from build123d import *

# Parameters (mm, degrees)
F1_DEPTH = 609.6
F3_D     = 25.4


with BuildPart() as f1:
    # F0 (on Top) → F1 (new body)
    with BuildSketch(Plane.XY):
        with BuildLine():
            ThreePointArc((38.1, 25.4), (34.380256, 34.380256), (25.4, 38.1))
            Line((25.4, 38.1), (-25.4, 38.1))
            ThreePointArc((-25.4, 38.1), (-34.380256, 34.380256), (-38.1, 25.4))
            Line((-38.1, 25.4), (-38.1, -25.4))
            ThreePointArc((-38.1, -25.4), (-34.380256, -34.380256), (-25.4, -38.1))
            Line((-25.4, -38.1), (25.4, -38.1))
            ThreePointArc((25.4, -38.1), (34.380256, -34.380256), (38.1, -25.4))
            Line((38.1, -25.4), (38.1, 25.4))
        make_face()
        with BuildLine():
            ThreePointArc((25.4, 33.3375), (31.01266, 31.01266), (33.3375, 25.4))
            Line((33.3375, 25.4), (33.3375, -25.4))
            ThreePointArc((33.3375, -25.4), (31.01266, -31.01266), (25.4, -33.3375))
            Line((25.4, -33.3375), (-25.4, -33.3375))
            ThreePointArc((-25.4, -33.3375), (-31.01266, -31.01266), (-33.3375, -25.4))
            Line((-33.3375, -25.4), (-33.3375, 25.4))
            ThreePointArc((-33.3375, 25.4), (-31.01266, 31.01266), (-25.4, 33.3375))
            Line((-25.4, 33.3375), (25.4, 33.3375))
        make_face(mode=Mode.SUBTRACT)
    extrude(amount=F1_DEPTH)

    # F3 (through all)
    with Locations(Plane.YZ.offset(38.1)):
        with Locations((0, 571.5), (0, 38.1)):
            Hole(F3_D / 2)


solid = f1.part
Here's how the part is built. I have some questions about the finished solid (model axes, mm). A direction names the side the tool comes from. Coordinates: 2 decimals unless noted, no trailing zeros. Loops run counter-clockwise (first coordinate to the right, second up) from the corner with the lowest first, then second, coordinate; pieces in that order, holes last. Notation, with made-up numbers: (-21.75, 48.5) -> (37.25, 48.5) arc R13 cw to (37.25, 61.5) -> close; hole circle Ø6 at (-24, 85). An arc over 180 degrees is marked (long way). Use one line per item in the form item = value. Start each with the question number.
(1) If we section it at B-B (z = 334): Please give me the cut outline in (x, y) (1 decimal).
(2) If we section it at D-D (z = 571.5): Please give me the cut outline in (x, y) (1 decimal), then the cut area to 3 significant figures.
(3) Will this pin go through, and if not, where does the flat tip stop? pin 1 (23 mm diameter, centred on y = 0, z = 38.1, fed in from +X).
(4) On a 3-axis mill with a long thin cutter (end or side, diameter ignored), from which of +Z, -Z, +X, -X, +Y, -Y can I reach the whole of each face in a straight line? I mean faces 1 (the face through (38.1, 0, 301)), 2 (the face through (0, 33.338, 301)). Say none if no direction works.
(5) Please list where these lines run through material, in increasing order: line 1 along Z through (x, y) = (-36, 0); line 2 along Y through (x, z) = (2.5, 554.5).
(6) If we section it at C-C (x = 14): Please give me the cut outline in (y, z), then the cut area to 3 significant figures.
(7) We'd pull the mould along Y, two halves only. Please class faces 3 (the face through (-3, 34, 609.6)), 4 (the face through (34.28, -34.48, 300.53)), 5 (the face through (33.338, 0, 301)): pulls with the +Y half, pulls with the -Y half, needs draft (parallel to the pull), parting line crosses it, or undercut.
(8) If we section it at A-A (y = 0): Please give me the cut outline in (x, z).
Verdict:
q1.outline = (-38.1, -25.4) arc R12.7 ccw to (-25.4, -38.1) -> (25.4, -38.1) arc R12.7 ccw to (38.1, -25.4) -> (38.1, 25.4) arc R12.7 ccw to (25.4, 38.1) -> (-25.4, 38.1) arc R12.7 ccw to (-38.1, 25.4) -> close; hole (-33.3, -25.4) arc R7.9 ccw to (-25.4, -33.3) -> (25.4, -33.3) arc R7.9 ccw to (33.3, -25.4) -> (33.3, 25.4) arc R7.9 ccw to (25.4, 33.3) -> (-25.4, 33.3) arc R7.9 ccw to (-33.3, 25.4) -> close
q2.outline = (-38.1, -25.4) arc R12.7 ccw to (-25.4, -38.1) -> (25.4, -38.1) arc R12.7 ccw to (38.1, -25.4) -> (38.1, -12.7) -> (33.3, -12.7) -> (33.3, -25.4) arc R7.9 cw to (25.4, -33.3) -> (-25.4, -33.3) arc R7.9 cw to (-33.3, -25.4) -> (-33.3, -12.7) -> (-38.1, -12.7) -> close; (-38.1, 12.7) -> (-33.3, 12.7) -> (-33.3, 25.4) arc R7.9 cw to (-25.4, 33.3) -> (25.4, 33.3) arc R7.9 cw to (33.3, 25.4) -> (33.3, 12.7) -> (38.1, 12.7) -> (38.1, 25.4) arc R12.7 ccw to (25.4, 38.1) -> (-25.4, 38.1) arc R12.7 ccw to (-38.1, 25.4) -> close
q2.area = 1,030 mm²
q3.pin_1 = through
q4.face_1 = +Z, -Z, +X, +Y, -Y
q4.face_2 = +Z, -Z
q5.line_1 = 0 to 25.4, 50.8 to 558.8, 584.2 to 609.6
q5.line_2 = -38.1 to -33.34, 33.34 to 38.1
q6.outline = (-38.1, 0) -> (-33.34, 0) -> (-33.34, 609.6) -> (-38.1, 609.6) -> close; (33.34, 0) -> (38.1, 0) -> (38.1, 609.6) -> (33.34, 609.6) -> close
q6.area = 5,810 mm²
q7.face_3 = needs draft
q7.face_4 = pulls with the -Y half
q7.face_5 = undercut
q8.outline = (-38.1, 0) -> (-33.34, 0) -> (-33.34, 25.4) -> (-38.1, 25.4) -> close; (-38.1, 50.8) -> (-33.34, 50.8) -> (-33.34, 558.8) -> (-38.1, 558.8) -> close; (-38.1, 584.2) -> (-33.34, 584.2) -> (-33.34, 609.6) -> (-38.1, 609.6) -> close; (33.34, 0) -> (38.1, 0) -> (38.1, 25.4) -> (33.34, 25.4) -> close; (33.34, 50.8) -> (38.1, 50.8) -> (38.1, 558.8) -> (33.34, 558.8) -> close; (33.34, 584.2) -> (38.1, 584.2) -> (38.1, 609.6) -> (33.34, 609.6) -> close
